```python
from build123d import *

# Parameters (mm, degrees)
SKETCH1_R           = 2.5
BOSS_EXTRUDE1_DEPTH = 10
SKETCH2_R           = 30.5
SKETCH2_R_2         = 19.5
CUT_EXTRUDE1_DEPTH  = 4
SKETCH3_R           = 17.5
BOSS_EXTRUDE2_DEPTH = 30
CUT_EXTRUDE2_DEPTH  = 10
FILLET1_R           = 10
SKETCH9_R           = 2.5
CUT_EXTRUDE4_DEPTH  = 20
BOSS_EXTRUDE3_START = 7.38
SKETCH10_R          = 7.5
SKETCH10_R_2        = 2.5
BOSS_EXTRUDE3_DEPTH = 7.38
CHAMFER1_SIZE       = 2


with BuildPart() as part:
    # Sketch1 → Boss-Extrude1 (new body)
    with BuildSketch(Plane(origin=(0, 0, 0), x_dir=(1, 0, 0), z_dir=(0, 1, 0))):
        with BuildLine():
            Line((-99.5, 86.5), (99.5, 86.5))
            ThreePointArc((99.5, 86.5), (107.985281374, 82.985281374), (111.5, 74.5))
            Line((111.5, 74.5), (111.5, -74.5))
            ThreePointArc((111.5, -74.5), (107.985281374, -82.985281374), (99.5, -86.5))
            Line((99.5, -86.5), (-99.5, -86.5))
            ThreePointArc((-99.5, -86.5), (-107.985281374, -82.985281374), (-111.5, -74.5))
            Line((-111.5, -74.5), (-111.5, 74.5))
            ThreePointArc((-111.5, 74.5), (-107.985281374, 82.985281374), (-99.5, 86.5))
        make_face()
        with Locations(Location((100, 75, 0), (0, 0, 270))):
            Circle(SKETCH1_R, mode=Mode.SUBTRACT)
        with Locations(Location((100, -75, 0), (0, 0, 270))):
            Circle(SKETCH1_R, mode=Mode.SUBTRACT)
        with Locations(Location((-100, -75, 0), (0, 0, 270))):
            Circle(SKETCH1_R, mode=Mode.SUBTRACT)
        with Locations(Location((-100, 75, 0), (0, 0, 270))):
            Circle(SKETCH1_R, mode=Mode.SUBTRACT)
    extrude(amount=-BOSS_EXTRUDE1_DEPTH)

    # Sketch2 → Cut-Extrude1 (cut)
    with BuildSketch(Plane(origin=(0, 0, 0), x_dir=(1, 0, 0), z_dir=(0, 1, 0))):
        with Locations(Location((0, 0, 0), (0, 0, 270))):
            Circle(SKETCH2_R)
        with Locations(Location((0, 0, 0), (0, 0, 270))):
            Circle(SKETCH2_R_2, mode=Mode.SUBTRACT)
    extrude(amount=-CUT_EXTRUDE1_DEPTH, mode=Mode.SUBTRACT)

    # Sketch3 → Boss-Extrude2 (add)
    with BuildSketch(Plane(origin=(0, 0, 0), x_dir=(1, 0, 0), z_dir=(0, 1, 0))):
        with Locations(Location((0, 0, 0), (0, 0, 270))):
            Circle(SKETCH3_R)
    extrude(amount=BOSS_EXTRUDE2_DEPTH)

    # Sketch6 → Cut-Extrude2 (cut, symmetric)
    with BuildSketch(Plane(origin=(0, 0, 0), x_dir=(0, 0, -1), z_dir=(1, 0, 0))):
        Polygon((-10, 30), (10, 30), (10, -10), (-10, -10), (-17.5, -10), (-10, -2.5), align=None)
    extrude(amount=CUT_EXTRUDE2_DEPTH, both=True, mode=Mode.SUBTRACT)

    # Fillet1
    fillet1_edges = [part.edges().sort_by_distance(p)[0] for p in [
        (10, 13.75, 10),
        (-10, 13.75, 10),
        (-10, 10, -10),
        (10, 10, -10),
    ]]
    fillet(fillet1_edges, radius=FILLET1_R - 0.0001)  # a hair under: the kernel refuses the full size

    # Sketch9 → Cut-Extrude4 (cut)
    with BuildSketch(Plane(origin=(0, 0, 0), x_dir=(1, 0, 0), z_dir=(0, 1, 0))):
        with Locations(Location((41, 71.01408311, 0), (0, 0, 270))):
            Circle(SKETCH9_R)
        with Locations(Location((82, 0, 0), (0, 0, 270))):
            Circle(SKETCH9_R)
        with Locations(Location((41, -71.01408311, 0), (0, 0, 270))):
            Circle(SKETCH9_R)
        with Locations(Location((-41, -71.01408311, 0), (0, 0, 270))):
            Circle(SKETCH9_R)
        with Locations(Location((-82, 0, 0), (0, 0, 270))):
            Circle(SKETCH9_R)
        with Locations(Location((-41, 71.01408311, 0), (0, 0, 270))):
            Circle(SKETCH9_R)
    extrude(amount=-CUT_EXTRUDE4_DEPTH, mode=Mode.SUBTRACT)

    # Sketch10 → Boss-Extrude3 (add)
    # profile 1 of 6: a face of its own
    with BuildSketch(Plane(origin=(0, 0, 0), x_dir=(1, 0, 0), z_dir=(0, 1, 0)).offset(BOSS_EXTRUDE3_START)):
        with Locations(Location((41, 71.01408311, 0), (0, 0, 270))):
            Circle(SKETCH10_R)
        with Locations(Location((41, 71.01408311, 0), (0, 0, 270))):
            Circle(SKETCH10_R_2, mode=Mode.SUBTRACT)
    # profile 2 of 6: a face of its own
    with BuildSketch(Plane(origin=(0, 0, 0), x_dir=(1, 0, 0), z_dir=(0, 1, 0)).offset(BOSS_EXTRUDE3_START)):
        with Locations(Location((82, 0, 0), (0, 0, 270))):
            Circle(SKETCH10_R)
        with Locations(Location((82, 0, 0), (0, 0, 270))):
            Circle(SKETCH10_R_2, mode=Mode.SUBTRACT)
    # profile 3 of 6: a face of its own
    with BuildSketch(Plane(origin=(0, 0, 0), x_dir=(1, 0, 0), z_dir=(0, 1, 0)).offset(BOSS_EXTRUDE3_START)):
        with Locations(Location((41, -71.01408311, 0), (0, 0, 270))):
            Circle(SKETCH10_R)
        with Locations(Location((41, -71.01408311, 0), (0, 0, 270))):
            Circle(SKETCH10_R_2, mode=Mode.SUBTRACT)
    # profile 4 of 6: a face of its own
    with BuildSketch(Plane(origin=(0, 0, 0), x_dir=(1, 0, 0), z_dir=(0, 1, 0)).offset(BOSS_EXTRUDE3_START)):
        with Locations(Location((-41, -71.01408311, 0), (0, 0, 270))):
            Circle(SKETCH10_R)
        with Locations(Location((-41, -71.01408311, 0), (0, 0, 270))):
            Circle(SKETCH10_R_2, mode=Mode.SUBTRACT)
    # profile 5 of 6: a face of its own
    with BuildSketch(Plane(origin=(0, 0, 0), x_dir=(1, 0, 0), z_dir=(0, 1, 0)).offset(BOSS_EXTRUDE3_START)):
        with Locations(Location((-82, 0, 0), (0, 0, 270))):
            Circle(SKETCH10_R)
        with Locations(Location((-82, 0, 0), (0, 0, 270))):
            Circle(SKETCH10_R_2, mode=Mode.SUBTRACT)
    # profile 6 of 6: a face of its own
    with BuildSketch(Plane(origin=(0, 0, 0), x_dir=(1, 0, 0), z_dir=(0, 1, 0)).offset(BOSS_EXTRUDE3_START)):
        with Locations(Location((-41, 71.01408311, 0), (0, 0, 270))):
            Circle(SKETCH10_R)
        with Locations(Location((-41, 71.01408311, 0), (0, 0, 270))):
            Circle(SKETCH10_R_2, mode=Mode.SUBTRACT)
    extrude(amount=-BOSS_EXTRUDE3_DEPTH)

    # Chamfer1
    chamfer1_edges = [part.edges().sort_by_distance(p)[0] for p in [
        (41, 7.38, -78.51408311),
        (82, 7.38, -7.5),
        (41, 7.38, 63.51408311),
        (41, 7.38, 68.51408311),
        (-41, 7.38, 63.51408311),
        (-82, 7.38, -7.5),
        (-41, 7.38, -78.51408311),
    ]]
    chamfer(chamfer1_edges, length=CHAMFER1_SIZE)


solid = part.part
```
Build history of the part. All positions in model axes, mm. A direction names the side the tool comes from. Round coordinates to 2 decimals unless told otherwise and drop trailing zeros. Loops run counter-clockwise (first coordinate to the right, second up) from the corner with the lowest first, then second, coordinate; pieces in that order, holes last.
Item 1: Saw through at D-D (x = -41). List the corners of the cut face in (y, z).
Item 2: Pin check, flat tips, straight feed: P1, Ø5, axis at x = -66.5, z = -8, coming from the +Y side; P2, Ø5.5, axis at x = 41, z = -70, coming from the +Y side; P3, Ø9, axis at y = 19.5, z = 5, coming from the -X side. Stop position of each tip, or through.
Item 3: Saw through at A-A (x = 41). List the corners of the cut face in (y, z).
Item 4: Saw through at C-C (x = 82). List the corners of the cut face in (y, z).
Item 5: Two-plate mould, pull along Z, no slides. Class faces 4 (the face through (-7.15, 13.98, 6.99)), 5 (the face through (-79, 7.38, 0)), 6 (the face through (107.89, -4.93, -83.08)): released by +Z, released by -Z, zero draft, split by the parting line, or undercut.
Item 6: Drill centre lines: line 1 along X through (y, z) = (-2.7, 0); line 2 along X through (y, z) = (-7, -75); line 3 along Y through (x, z) = (-67.5, -43). Where is each one in solid material? Low to high.
Item 7: Which spindle directions (+Z, -Z, +X, -X, +Y, -Y) get a long thin tool onto all of the face, cutting with end or side? Do faces 1 (the face through (-10, -5, 6)), 2 (the face through (-7.15, 9.72, -6.99)), 3 (the face through (-45.56, 2.73, 65.06)). Say none if no direction does.
Worked answers:
1. outline: (-10, -86.5) - (0, -86.5) - (0, -78.51) - (5.38, -78.51) - (7.38, -76.51) - (7.38, -73.51) - (-10, -73.51) - close; (-10, -68.51) - (7.38, -68.51) - (7.38, -65.51) - (5.38, -63.51) - (0, -63.51) - (0, 63.51) - (5.38, 63.51) - (7.38, 65.51) - (7.38, 68.51) - (-10, 68.51) - close; (-10, 73.51) - (7.38, 73.51) - (7.38, 76.51) - (5.38, 78.51) - (0, 78.51) - (0, 86.5) - (-10, 86.5) - close
2. P1: stops at y = 0
2. P2: stops at y = 7.38
2. P3: stops at x = -17.49
3. outline: (-10, -86.5) - (0, -86.5) - (0, -78.51) - (5.38, -78.51) - (7.38, -76.51) - (7.38, -73.51) - (-10, -73.51) - close; (-10, -68.51) - (7.38, -68.51) - (7.38, -65.51) - (5.38, -63.51) - (0, -63.51) - (0, 63.51) - (5.38, 63.51) - (7.38, 65.51) - (7.38, 66.51) - (5.38, 68.51) - (-10, 68.51) - close; (-10, 73.51) - (5.38, 73.51) - (7.38, 75.51) - (7.38, 76.51) - (5.38, 78.51) - (0, 78.51) - (0, 86.5) - (-10, 86.5) - close
4. outline: (-10, -86.5) - (0, -86.5) - (0, -7.5) - (5.38, -7.5) - (7.38, -5.5) - (7.38, -2.5) - (-10, -2.5) - close; (-10, 2.5) - (7.38, 2.5) - (7.38, 5.5) - (5.38, 7.5) - (0, 7.5) - (0, 86.5) - (-10, 86.5) - close
5. face 4: undercut
5. face 5: zero draft
5. face 6: released by -Z
6. line 1: x = -111.5 to -84.5, -79.5 to -30.5, -19.5 to -10, 10 to 19.5, 30.5 to 79.5, 84.5 to 111.5
6. line 2: x = -111.49 to -102.5, -97.5 to 97.5, 102.5 to 111.49
6. line 3: y = -10 to 0
7. face 1: -Y
7. face 2: +Y, -Y
7. face 3: +Y
